from build123d import *

# Parameters (mm, degrees)
SKETCH_1_R          = 5
EXTRUDE_1_DEPTH     = 10
SKETCH_1_3_W        = 10
SKETCH_1_3_H        = 5
EXTRUDE_2_DEPTH     = 15
SKETCH_1_4_W        = 5
SKETCH_1_4_H        = 20
EXTRUDE_3_DEPTH     = 20
CUT_EXTRUDE_1_DEPTH = 20


with BuildPart() as part:
    # Sketch 1 → Extrude 1 (new body)
    with BuildSketch(Plane(origin=(0, 0, 0), x_dir=(1, 0, 0), z_dir=(0, 1, 0))):
        Polygon((10, 15), (5, 15), (5, 10), (-5, 10), (-10, 10), (-10, -10), (10, -10), align=None)
        Circle(SKETCH_1_R, mode=Mode.SUBTRACT)
    extrude(amount=EXTRUDE_1_DEPTH)

    # Sketch 1_3 → Extrude 2 (add)
    with BuildSketch(Plane(origin=(0, 0, 0), x_dir=(1, 0, 0), z_dir=(0, 1, 0))):
        with Locations((0, 12.5)):
            Rectangle(SKETCH_1_3_W, SKETCH_1_3_H)
    extrude(amount=EXTRUDE_2_DEPTH)

    # Sketch 1_4 → Extrude 3 (add)
    with BuildSketch(Plane(origin=(0, 0, 0), x_dir=(1, 0, 0), z_dir=(0, 1, 0))):
        Polygon((-5, 15), (-15, 15), (-15, 10), (-10, 10), (-5, 10), align=None)
        with Locations((-12.5, 0)):
            Rectangle(SKETCH_1_4_W, SKETCH_1_4_H)
    extrude(amount=EXTRUDE_3_DEPTH)

    # Sketch 2 → Cut-Extrude 1 (cut)
    with BuildSketch(Plane(origin=(-10, 0, 0), x_dir=(0, 0, -1), z_dir=(1, 0, 0))):
        Polygon((-10, 10), (10, 20), (-10, 20), align=None)
    extrude(amount=-CUT_EXTRUDE_1_DEPTH, mode=Mode.SUBTRACT)


solid = part.part
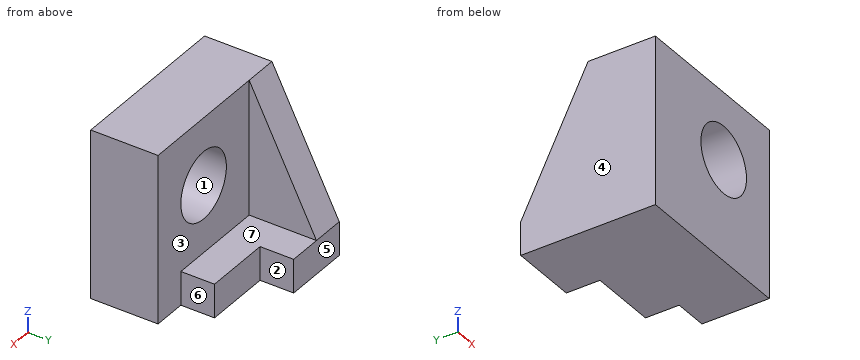
Check sheet for the modelled part. Datum: model origin and axes. Units: mm. Face numbers are marked on the shaded views. A direction names the side the tool comes from. Coordinates: 2 decimals unless noted, no trailing zeros. Write each loop counter-clockwise with the first axis right and the second up, starting at its lowest first coordinate (ties: lowest second). Pieces come first, ordered by that corner, then holes.
Item 1: Cross-section at A-A on z = 0. Record the boundary of the cut face in (x, y).
Numbers:
outline: (-15, 0) - (-5, 0) - (-5, 10) - (-10, 10) - (-10, 15) - (-15, 15) - close; (5, 0) - (10, 0) - (10, 10) - (5, 10) - close
Item 2: Scan lines: probe 1 along X at (y, z) = (3.75, 0); probe 2 along Y at (x, z) = (4, -4.75). Record each from-to range of solid material in increasing order.
Numbers:
probe 1: x = -15 to -5, 5 to 10
probe 2: y = 0 to 10
Item 3: Cross-section at B-B on x = 0. Record the boundary of the cut face in (y, z).
Numbers:
outline: (0, -15) - (15, -15) - (15, -10) - (10, -10) - (10, -5) - (0, -5) - close; (0, 5) - (10, 5) - (10, 10) - (0, 10) - close
Item 4: Mould release check, pull along X, two halves, no side actions. Record for the marked faces 1, 2, 3 and 4: released by +X, released by -X, zero draft, split by the parting line, or undercut.
Numbers:
face 1: undercut
face 2: released by +X
face 3: zero draft
face 4: released by -X
Item 5: Cross-section at C-C on y = 5.25. Record the boundary of the cut face in (x, z), then the cut area to 3 significant figures.
Numbers:
outline: (-15, -15) - (10, -15) - (10, 10) - (-15, 10) - close; hole circle Ø10 at (0, 0)
area: 546 mm2
Item 6: Cross-section at D-D on z = -12.5. Record the boundary of the cut face in (x, y), then the cut area to 3 significant figures.
Numbers:
outline: (-15, 0) - (10, 0) - (10, 10) - (5, 10) - (5, 15) - (-5, 15) - (-5, 20) - (-15, 20) - close
area: 400 mm2
Item 7: Access from +Z, -Z, +X, -X, +Y, -Y to the whole of each face (thin tool, end or side, straight path). Record for the marked faces 5, 6 and 7.
Numbers:
face 5: +Z, -Z, +X, -X, +Y
face 6: +Z, -Z, +X, +Y
face 7: +Z, +X, +Y
Item 8: Depth check by flat-ended pin: pin 1 Ø5.5 at (y, z) = (17, -11.5) entering from +X; pin 2 Ø2.5 at (x, z) = (-1, -13.5) entering from +Y; pin 3 Ø5 at (y, z) = (15, -2.5) entering from +X. Enter the tip coordinate at first touch or a pass-through.
Numbers:
pin 1: stops at x = 5
pin 2: stops at y = 15
pin 3: stops at x = -10
